Design review of the part built by this model. Coordinates are the model's own, in mm. Face numbers are marked on the shaded views. Coordinates: 2 decimals unless noted, no trailing zeros. Order: outer loops, then holes, each group sorted by start corner. A loop starts at its lowest first (then second) coordinate and runs counter-clockwise, first axis right, second up. Notation, with made-up numbers: M 55,22 L 86,22 A14 ccw 86,49 Z; hole C 27.25,28.25 d1. An arc over 180 degrees is marked long. Answer as a JSON object with one key per item and string values.
from build123d import *

# Parameters (mm, degrees)
F0_W            = 4.7625
F0_H            = 12.7
F3_R            = 1.143
F4_DEPTH        = 12.7
F4_COPIES_COUNT = 7


# Not quite as in the source:
# - a pattern or mirror of a feature is missing from the dataset's text; its kind, count and spacing are read off the source's solid


with BuildPart() as f1:
    # F0 (on Top) → F1 (revolve)
    with BuildSketch(Plane.XY):
        with Locations((14.77645, 0)):
            Rectangle(F0_W, F0_H)
    revolve(axis=Axis((0, -1.5469156838, 0), (0, -1, 0)))

    # F3 (on face) → F4 (cut, through all)
    with BuildSketch(Plane.XZ.offset(6.35)):
        with Locations((0, 14.859)):
            Circle(F3_R)
    f4 = extrude(amount=-F4_DEPTH, mode=Mode.SUBTRACT)

    # F4_copies: F4 ×7 about axis
    f4_copies_axis = Axis((0, 0, 0), (0, 1, 0))
    for i in range(1, F4_COPIES_COUNT):
        add(f4.rotate(f4_copies_axis, i * 360 / F4_COPIES_COUNT), mode=Mode.SUBTRACT)


solid = f1.part
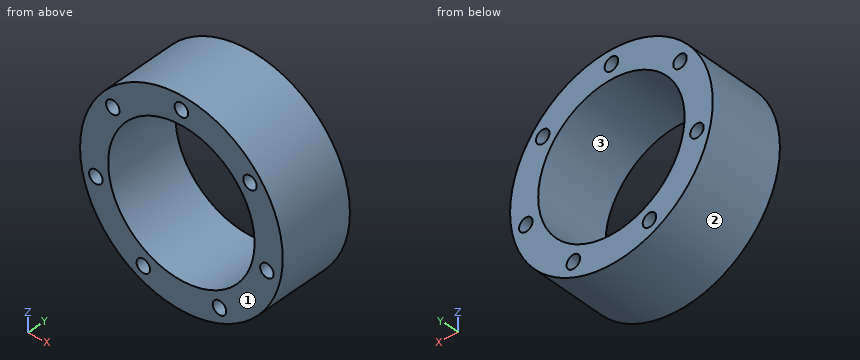
1) To check wall thickness, follow L1, parallel to Z at x = 0, y = -1.5; L2, parallel to X at y = -5.25, z = -2.5; L3, parallel to X at y = 4, z = 0.5. State the ranges of each line that lie inside material, in increasing order.
Taken from the geometry:
{"L1": "z = -17.16 to -12.4, 12.4 to 13.72, 16 to 17.16", "L2": "x = -16.97 to -15.3, -13.68 to -12.14, 12.14 to 13.68, 15.3 to 16.97", "L3": "x = -17.15 to -12.39, 12.39 to 17.15"}
2) Mouldability with a two-part tool opening along X and no side actions: class the marked faces 1, 2 and 3 as released by +X, released by -X, zero draft, split by the parting line, or undercut.
Taken from the geometry:
{"face 1": "zero draft", "face 2": "split by the parting line", "face 3": "undercut"}
3) Add section A-A (z = 0). State the section outline as (x, y) points, and give its area (3 significant figures).
Taken from the geometry:
{"outline": "M -17.16,-6.35 L -12.4,-6.35 L -12.4,6.35 L -17.16,6.35 Z; M 12.4,-6.35 L 17.16,-6.35 L 17.16,6.35 L 12.4,6.35 Z", "area": "121 mm2"}
4) Add section D-D (y = -5.5). Count the separate pieces of the cut face and the enclosed holes in it, and give its area (3 significant figures).
Taken from the geometry:
{"separate pieces": "1", "enclosed holes": "8", "area": "413 mm2"}
5) Add section B-B (x = 0). State the section outline as (y, z) points, and give its area (3 significant figures).
Taken from the geometry:
{"outline": "M -6.35,-17.16 L 6.35,-17.16 L 6.35,-12.4 L -6.35,-12.4 Z; M -6.35,12.4 L 6.35,12.4 L 6.35,13.72 L -6.35,13.72 Z; M -6.35,16 L 6.35,16 L 6.35,17.16 L -6.35,17.16 Z", "area": "91.9 mm2"}
6) Add section C-C (x = 9.5). State the section outline as (y, z) points, and give its area (3 significant figures).
Taken from the geometry:
{"outline": "M -6.35,-14.29 L 6.35,-14.29 L 6.35,-7.96 L -6.35,-7.96 Z; M -6.35,7.96 L 6.35,7.96 L 6.35,14.29 L -6.35,14.29 Z", "area": "161 mm2"}
7) Insertion check: pin 1 Ø2 at (x, z) = (14.49, -3.31) entering from -Y; pin 2 Ø5 at (x, y) = (-12.5, -0.5) entering from +Z; pin 3 Ø1.5 at (y, z) = (3.5, -8.5) entering from -X; pin 4 Ø6 at (y, z) = (-3.5, -9.5) entering from +X. Each pin has a flat end and moves straight along its axis. Give the tip position at first contact, or say it passes through.
Taken from the geometry:
{"pin 1": "passes through", "pin 2": "stops at z = 13.94", "pin 3": "stops at x = -15.31", "pin 4": "stops at x = 15.88"}
